```python
from build123d import *

# Parameters (mm, degrees)
F0_W     = 198.9582
F0_H     = 622.3
F0_W_2   = 221.1972716
F1_DEPTH = 88.9
F3_DEPTH = 698.5
F5_DEPTH = 698.501
F6_W     = 1482.6882716
F6_H     = 698.5
F7_DEPTH = 6.35
F8_W     = 1482.6882716
F8_H     = 698.5
F9_DEPTH = 6.35


# Not quite as in the source:
# - a feature names something its author has since deleted; it is built from what else it names


with BuildPart() as f1:
    # F0 (on Front) → F1 (new body)
    with BuildSketch(Plane.XZ):
        Polygon((0, 38.1), (0, 0), (1482.6882716, 0), (1482.6882716, 38.1), (1482.6882716, 660.4), (1482.6882716, 698.5), (0, 698.5), (0, 660.4), align=None)
        with Locations((137.5791, 349.25)):
            Rectangle(F0_W, F0_H, mode=Mode.SUBTRACT)
        with Locations((374.6373, 349.25)):
            Rectangle(F0_W, F0_H, mode=Mode.SUBTRACT)
        with Locations((611.6955, 349.25)):
            Rectangle(F0_W, F0_H, mode=Mode.SUBTRACT)
        with Locations((848.7537, 349.25)):
            Rectangle(F0_W, F0_H, mode=Mode.SUBTRACT)
        with Locations((1085.8119, 349.25)):
            Rectangle(F0_W, F0_H, mode=Mode.SUBTRACT)
        with Locations((1333.9896358, 349.25)):
            Rectangle(F0_W_2, F0_H, mode=Mode.SUBTRACT)
    extrude(amount=F1_DEPTH)

    # F2 (on face) → F3 (join, through all)
    with BuildSketch(Plane.XY.offset(698.5)):
        Polygon((-15.675468585, 0), (0, -88.9), (0, 0), align=None)
    extrude(amount=-F3_DEPTH)

    # F4 (on face) → F5 (cut, through all)
    with BuildSketch(Plane.XY.offset(698.5)):
        Polygon((1467.012803015, 0), (1482.6882716, -88.9), (1482.6882716, 0), align=None)
    extrude(amount=-F5_DEPTH, mode=Mode.SUBTRACT)

    # F6 (on face) → F7 (join)
    with BuildSketch(Plane.XZ.offset(88.9)):
        with Locations((741.3441358, 349.25)):
            Rectangle(F6_W, F6_H)
    extrude(amount=F7_DEPTH)

    # F8 (on face) → F9 (join)
    with BuildSketch(Plane(origin=(0, 0, 0), x_dir=(-1, 0, 0), z_dir=(0, 1, 0))):
        with Locations((-725.668667215, 349.25)):
            Rectangle(F8_W, F8_H)
    extrude(amount=F9_DEPTH)


solid = f1.part
```
CAD build for the part. Positions are in the model's coordinates, mm. A direction names the side the tool comes from. Round coordinates to 2 decimals unless told otherwise and drop trailing zeros. Order: outer loops, then holes, each group sorted by start corner. A loop starts at its lowest first (then second) coordinate and runs counter-clockwise, first axis right, second up.
Q1. Slice it at C-C (y = -37). Write the cut outline in (x, z).
Q2. Slice it at A-A (z = 367). State how many separate pieces and enclosed holes the cut face has, and give its area (3 significant figures).
Q3. Two-plate mould, pull along X, no slides. Class faces 1 (the flat face through (744, -45, 0)), 2 (the flat face through (376, 0, 354)), 3 (the flat face through (-7.947, -43.828, 354.14)), 4 (the flat face through (610, -88.9, 354)): pulls with the +X half, pulls with the -X half, needs draft (parallel to the pull), parting line crosses it, or undercut.
Q4. Drop flat-ended pins along their axis: pin 1 (5 mm diameter, centred on y = -24, z = 72, fed in from +X); pin 2 (4 mm diameter, centred on y = -76.5, z = 572, fed in from +X). Give the stop position or say it passes through.
Q5. Which spindle directions (+Z, -Z, +X, -X, +Y, -Y) get a long thin tool onto all of the face, cutting with end or side? Do faces 5 (the flat face through (1474.74, -43.83, 354.14)), 6 (the flat face through (847, -44, 38.1)). Say none if no direction does.
Q6. Wall check: L1, parallel to Y at x = 1174, z = 256; L2, parallel to Z at x = 900, y = -37.5. Give the ranges that are in metal, low to high.
Q7. Slice it at B-B (x = 125.5). Write the cut outline in (y, z).
Results below:
1. outline: (-9.15, 0) - (1473.54, 0) - (1473.54, 698.5) - (-9.15, 698.5) - close; hole (38.1, 38.1) - (237.06, 38.1) - (237.06, 660.4) - (38.1, 660.4) - close; hole (275.16, 38.1) - (474.12, 38.1) - (474.12, 660.4) - (275.16, 660.4) - close; hole (512.22, 38.1) - (711.17, 38.1) - (711.17, 660.4) - (512.22, 660.4) - close; hole (749.27, 38.1) - (948.23, 38.1) - (948.23, 660.4) - (749.27, 660.4) - close; hole (986.33, 38.1) - (1185.29, 38.1) - (1185.29, 660.4) - (986.33, 660.4) - close; hole (1223.39, 38.1) - (1444.59, 38.1) - (1444.59, 660.4) - (1223.39, 660.4) - close
2. separate pieces: 1
2. enclosed holes: 6
2. area: 42,500 mm2
3. face 1: needs draft
3. face 2: undercut
3. face 3: pulls with the -X half
3. face 4: undercut
4. pin 1: stops at x = 1471.69
4. pin 2: stops at x = 1480.85
5. face 5: +Z, -Z, +X, +Y
5. face 6: none
6. L1: y = -95.25 to -88.9, 0 to 6.35
6. L2: z = 0 to 38.1, 660.4 to 698.5
7. outline: (-95.25, 0) - (6.35, 0) - (6.35, 698.5) - (-95.25, 698.5) - close; hole (-88.9, 38.1) - (0, 38.1) - (0, 660.4) - (-88.9, 660.4) - close
